Geometry: final body of the model. Coordinates: model frame, mm. Give positions to 0.01 mm unless a question says otherwise; leave off trailing zeros. Write each loop counter-clockwise with the first axis right and the second up, starting at its lowest first coordinate (ties: lowest second). Pieces come first, ordered by that corner, then holes. Notation, with made-up numbers: (40, 5.5) - (91, 5.5) arc R32 cw to (91, 40.5) - close; hole circle Ø5 at (-30, 1.5). An arc over 180 degrees is marked (long way). Use CSV: the item, a comma, the result in double quotes. Start each with the question number.
(1) Section B-B on x = -193. Output: boundary loops of the cut face in (y, z), and give its area (3 significant figures).
(2) Section A-A on y = -1. Output: boundary loops of the cut face in (x, z).
(3) Line query: probe 1 along Z at (x, y) = (-122.5, -0.45); probe 2 along X at (y, z) = (-2.8, -29.5); probe 3 along Z at (x, y) = (-94.5, -2.8). Output: solid intervals per line, ascending. Write a range as [from, to].
(4) First-contact query: pin 1 Ø1.5 at (x, z) = (-51, 77) entering from +Y; pin 2 Ø0.9 at (y, z) = (-2, 93.5) entering from -X; pin 3 Ø1.5 at (x, y) = (-174.5, -1.5) entering from +Z; pin 4 Ø0.9 at (y, z) = (-1, 94) entering from +X. Flat tips, straight axial feed; report the tip coordinate or a pass-through.
from build123d import *

# Parameters (mm, degrees)
F0_W     = 8
F0_H     = 3.3
F1_DEPTH = 3


with BuildPart() as f1:
    # F0 (on Front) → F1 (new body)
    with BuildSketch(Plane.XZ):
        with BuildLine():
            Line((-220, -35.777669), (-220, -38.777669))
            Line((-220, -38.777669), (100, -38.777669))
            Line((100, -38.777669), (100, -35.777669))
            Line((100, -35.777669), (97, -35.777669))
            Line((97, -35.777669), (97, -25.444639))
            Line((97, -25.444639), (100, -25.444669))
            Line((100, -25.444669), (100, 91.222331))
            Line((100, 91.222331), (-19.945289, 91.222331))
            Line((-19.945289, 91.222331), (-19.945289, 96.801867))
            ThreePointArc((-19.945289, 96.801867), (-21.702648, 101.044508), (-25.945289, 102.801867))
            Line((-25.945289, 102.801867), (-94.054711, 102.801867))
            ThreePointArc((-94.054711, 102.801867), (-98.297352, 101.044508), (-100.054711, 96.801867))
            Line((-100.054711, 96.801867), (-100.054711, 91.222331))
            Line((-100.054711, 91.222331), (-220, 91.222331))
            Line((-220, 91.222331), (-220, -25.444669))
            Line((-220, -25.444669), (-217, -25.444669))
            Line((-217, -25.444669), (-217, -35.777669))
            Line((-217, -35.777669), (-220, -35.777669))
        make_face()
        with Locations((-74.548644, 89.151867)):
            Rectangle(F0_W, F0_H, mode=Mode.SUBTRACT)
        with Locations((-46.439216, 89.151867)):
            Rectangle(F0_W, F0_H, mode=Mode.SUBTRACT)
    extrude(amount=F1_DEPTH)


solid = f1.part
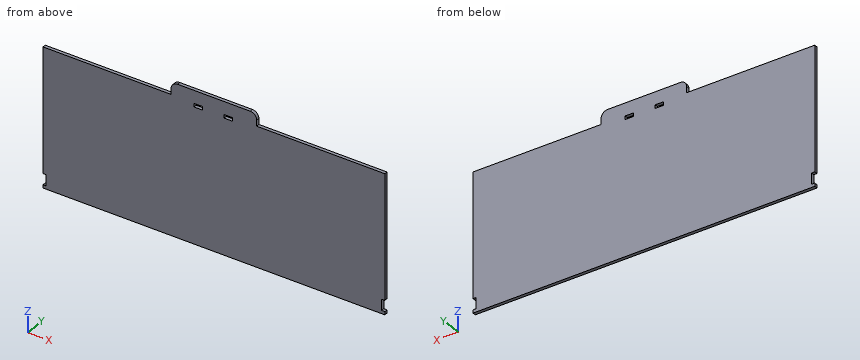
Check values:
1,outline,"(-3, -38.78) - (0, -38.78) - (0, 91.22) - (-3, 91.22) - close"
1,area,"390 mm²"
2,outline,"(-220, -38.78) - (100, -38.78) - (100, -35.78) - (97, -35.78) - (97, -25.44) - (100, -25.44) - (100, 91.22) - (-19.95, 91.22) - (-19.95, 96.8) arc R6 ccw to (-25.95, 102.8) - (-94.05, 102.8) arc R6 ccw to (-100.05, 96.8) - (-100.05, 91.22) - (-220, 91.22) - (-220, -25.44) - (-217, -25.44) - (-217, -35.78) - (-220, -35.78) - close; hole (-78.55, 87.5) - (-70.55, 87.5) - (-70.55, 90.8) - (-78.55, 90.8) - close; hole (-50.44, 87.5) - (-42.44, 87.5) - (-42.44, 90.8) - (-50.44, 90.8) - close"
3,probe 1,"z = [-38.78, 91.22]"
3,probe 2,"x = [-217, 97]"
3,probe 3,"z = [-38.78, 102.79]"
4,pin 1,"stops at y = 0"
4,pin 2,"stops at x = -100.05"
4,pin 3,"stops at z = 91.22"
4,pin 4,"stops at x = -19.95"
